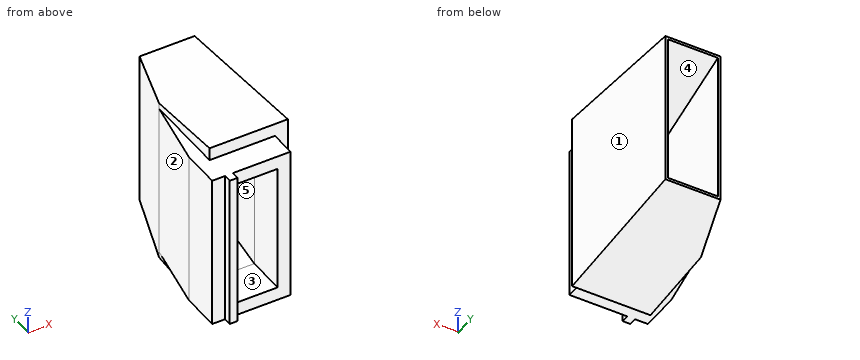
```python
from build123d import *

# Parameters (mm, degrees)
AUFSATZ_LINEAR_AUSTRAGEN1_DEPTH      = 60.4
AUFSATZ_LINEAR_AUSTRAGEN2_DEPTH      = 30.4
AUFSATZ_LINEAR_AUSTRAGEN3_DEPTH      = 55.2
AUFSATZ_LINEAR_AUSTRAGEN3_DEPTH_BACK = 5.2
SKIZZE4_W                            = 5
SKIZZE4_H                            = 10
SCHNITT_LINEAR_AUSTRAGEN1_DEPTH      = 66.4
SCHNITT_LINEAR_AUSTRAGEN4_DEPTH      = 6
SCHNITT_LINEAR_AUSTRAGEN4_DEPTH_BACK = 66.4


with BuildPart() as part:
    # Skizze1 → Aufsatz-Linear austragen1 (new body)
    with BuildSketch(Plane.XY):
        Polygon((14, 14.875), (14, 29.875), (23, 84.875), (24, 84.875), (24, 24.875), (19, 24.875), (19, 14.875), align=None)
    extrude(amount=AUFSATZ_LINEAR_AUSTRAGEN1_DEPTH)

    # Skizze2 → Aufsatz-Linear austragen2 (add)
    with BuildSketch(Plane(origin=(24, 0, 0), x_dir=(0, 0, -1), z_dir=(1, 0, 0))):
        Polygon((-59.4, 84.875), (-60.4, 84.875), (-65.4, 24.875), (-60.4, 24.875), (-60.4, 14.875), (-55.2, 14.875), (-55.2, 29.875), align=None)
        Polygon((0, 24.875), (0, 14.875), (-5.2, 14.875), (-5.2, 29.875), (-1, 84.875), (0, 84.875), (5, 24.875), align=None)
    extrude(amount=-AUFSATZ_LINEAR_AUSTRAGEN2_DEPTH)

    # Skizze3 → Aufsatz-Linear austragen3 (add, two sides)
    with BuildSketch(Plane.XY.offset(5.2)) as aufsatz_linear_austragen3_sk:
        Polygon((-3.4, 29.875), (-3.4, 14.875), (-3.4, 11.875), (-6.4, 11.875), (-6.4, 14.875), (-11.4, 14.875), (-11.4, 29.875), (-1.4, 84.875), (3.6, 84.875), align=None)
    extrude(amount=AUFSATZ_LINEAR_AUSTRAGEN3_DEPTH)
    extrude(aufsatz_linear_austragen3_sk.sketch, amount=-AUFSATZ_LINEAR_AUSTRAGEN3_DEPTH_BACK)

    # Skizze4 → Schnitt-Linear austragen1 (cut, through all)
    with BuildSketch(Plane.XY.offset(60.4)):
        with Locations((21.5, 19.875)):
            Rectangle(SKIZZE4_W, SKIZZE4_H)
    extrude(amount=-SCHNITT_LINEAR_AUSTRAGEN1_DEPTH, mode=Mode.SUBTRACT)

    # Skizze7 → Schnitt-Linear austragen4 (cut, two sides)
    with BuildSketch(Plane(origin=(0, 0, 0), x_dir=(-1, 0, 0), z_dir=(0, 0, -1))) as schnitt_linear_austragen4_sk:
        Polygon((6.4, 57.375), (-2.6, 84.875), (6.4, 84.875), align=None)
    extrude(amount=SCHNITT_LINEAR_AUSTRAGEN4_DEPTH, mode=Mode.SUBTRACT)
    extrude(schnitt_linear_austragen4_sk.sketch, amount=-SCHNITT_LINEAR_AUSTRAGEN4_DEPTH_BACK, mode=Mode.SUBTRACT)


solid = part.part
```
Build history of the part. All positions in model axes, mm. Face numbers are marked on the shaded views. A direction names the side the tool comes from. Coordinates: 2 decimals unless noted, no trailing zeros. Order: outer loops, then holes, each group sorted by start corner. A loop starts at its lowest first (then second) coordinate and runs counter-clockwise, first axis right, second up. Notation, with made-up numbers: (42, 48.25) -> (86, 48.25) arc R9 ccw to (86, 64.25) -> close; hole circle Ø11 at (1.25, 86). An arc over 180 degrees is marked (long way). Answer in a Markdown table with one row per item. Add a question column.
Q1. Wall check: line 1 along X through (y, z) = (26, 40.5); line 2 along Z through (x, y) = (1, 16); line 3 along X through (y, z) = (67.5, 32). Give the ranges that are in metal, low to high. Write a range as [from, to].
Q2. Band-saw the part on C-C, the plane y = 18.5. List the corners of the cut face in (x, z).
Q3. Band-saw the part on B-B, the plane x = 4.5. List the corners of the cut face in (y, z) (3 decimals).
Q4. Drop flat-ended pins along their axis: pin 1 (5 mm diameter, centred on x = 12, y = 56, fed in from -Z); pin 2 (12 mm diameter, centred on y = 53.5, z = 39.5, fed in from -X); pin 3 (16.5 mm diameter, centred on x = 6.5, y = 23, fed in from +Z). Give the stop position or say it passes through.
Q5. Mould opens along X. For the marked faces 1, 2 and 3 say: +X half, -X half, draft (parallel to the pull), parting line (faces both ways), or undercut.
Q6. Band-saw the part on A-A, the plane z = 30.5. List the corners of the cut face in (x, y) (3 decimals).
Q7. Which spindle directions (+Z, -Z, +X, -X, +Y, -Y) get a long thin tool onto all of the face, cutting with end or side? Do the marked faces 4 and 5. Say none if no direction does.
Q8. Band-saw the part on D-D, the plane z = 57. List the corners of the cut face in (x, y) (3 decimals).
Answers follow:
| question | item | result |
|---|---|---|
| 1 | line 1 | [-11.4, -3.4], [14, 24] |
| 1 | line 2 | [0, 5.2], [55.2, 60.4] |
| 1 | line 3 | [-3.09, 1.39], [20.16, 24] |
| 2 | outline | (-11.4, 0) -> (19, 0) -> (19, 60.4) -> (-11.4, 60.4) -> close; hole (-3.4, 5.2) -> (14, 5.2) -> (14, 55.2) -> (-3.4, 55.2) -> close |
| 3 | outline | (14.875, 0) -> (24.875, 0) -> (24.875, -5) -> (84.875, 0) -> (84.875, 1) -> (29.875, 5.2) -> (14.875, 5.2) -> close; (14.875, 55.2) -> (29.875, 55.2) -> (84.875, 59.4) -> (84.875, 60.4) -> (24.875, 65.4) -> (24.875, 60.4) -> (14.875, 60.4) -> close |
| 4 | pin 1 | z = -2.61 |
| 4 | pin 2 | x = -8.2 |
| 4 | pin 3 | z = 65.4 |
| 5 | face 1 | +X half |
| 5 | face 2 | -X half |
| 5 | face 3 | undercut |
| 6 | outline | (-11.4, 14.875) -> (-6.4, 14.875) -> (-6.4, 11.875) -> (-3.4, 11.875) -> (-3.4, 29.875) -> (3.6, 84.875) -> (2.6, 84.875) -> (-6.4, 57.375) -> (-11.4, 29.875) -> close; (14, 14.875) -> (19, 14.875) -> (19, 24.875) -> (24, 24.875) -> (24, 84.875) -> (23, 84.875) -> (14, 29.875) -> close |
| 7 | face 4 | none |
| 7 | face 5 | +Y |
| 8 | outline | (-11.4, 14.875) -> (-6.4, 14.875) -> (-6.4, 11.875) -> (-3.4, 11.875) -> (-3.4, 14.875) -> (19, 14.875) -> (19, 24.875) -> (24, 24.875) -> (24, 84.875) -> (23, 84.875) -> (17.857, 53.446) -> (-0.4, 53.446) -> (3.6, 84.875) -> (2.6, 84.875) -> (-6.4, 57.375) -> (-11.4, 29.875) -> close |
